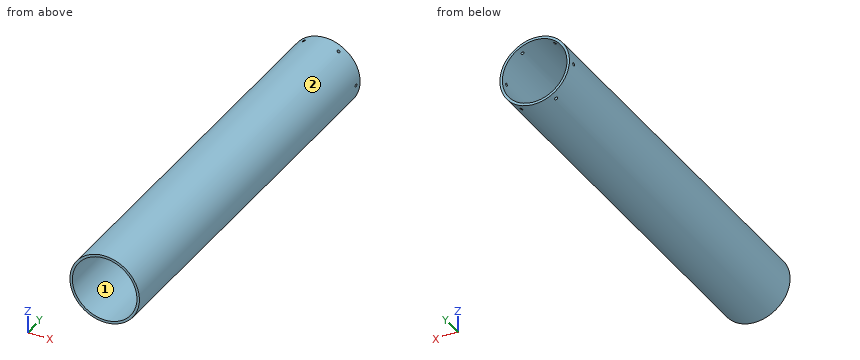
```python
from build123d import *

# Parameters (mm, degrees)
SKETCH1_R               = 70
SKETCH1_R_2             = 65
BOSS_EXTRUDE1_DEPTH     = 800
CUT_EXTRUDE1_REACH      = 808.102
CUT_EXTRUDE1_END_RADIUS = 70
SKETCH2_R               = 3.05
CIRPATTERN1_COUNT       = 6


with BuildPart() as part:
    # Sketch1 → Boss-Extrude1 (new body)
    with BuildSketch(Plane(origin=(0, 0, 0), x_dir=(1, 0, 0), z_dir=(0, 1, 0))):
        with Locations(Location((0, 0, 0), (0, 0, 270))):
            Circle(SKETCH1_R)
        with Locations(Location((0, 0, 0), (0, 0, 270))):
            Circle(SKETCH1_R_2, mode=Mode.SUBTRACT)
    extrude(amount=BOSS_EXTRUDE1_DEPTH)

    # Cut-Extrude1: up to this cylinder (the profile starts inside it)
    cut_extrude1_end = Plane(origin=(0, 785, 0), z_dir=(0, -1, 0)) * Cylinder(CUT_EXTRUDE1_END_RADIUS, 1757.204, mode=Mode.PRIVATE)
    # Sketch2 → Cut-Extrude1 (cut, up to the surface)
    with BuildSketch(Plane(origin=(0, 0, 0), x_dir=(0, 0, -1), z_dir=(1, 0, 0)), mode=Mode.PRIVATE) as cut_extrude1_sk1:
        with Locations((0, 785)):
            Circle(SKETCH2_R)
    cut_extrude1_tool1 = extrude(cut_extrude1_sk1.sketch, amount=-CUT_EXTRUDE1_REACH, mode=Mode.PRIVATE) & cut_extrude1_end
    cut_extrude1 = cut_extrude1_tool1.solids().sort_by_distance((0, 785, 0))[0]
    add(cut_extrude1, mode=Mode.SUBTRACT)

    # CirPattern1: Cut-Extrude1 ×6 about axis
    cirpattern1_axis = Axis((0, 800, 0), (0, 1, 0))
    for i in range(1, CIRPATTERN1_COUNT):
        add(cut_extrude1.rotate(cirpattern1_axis, i * 360 / CIRPATTERN1_COUNT), mode=Mode.SUBTRACT)


solid = part.part
```
Can you work these out from the model? Positions are in its coordinate system, mm. Face numbers are marked on the shaded views. Give positions to 0.01 mm unless a question says otherwise; leave off trailing zeros. Order: outer loops, then holes, each group sorted by start corner. A loop starts at its lowest first (then second) coordinate and runs counter-clockwise, first axis right, second up. Notation, with made-up numbers: M -1,25.25 L 15,25.25 A26 ccw 15,43.25 Z; hole C 32.25,11.25 d8. An arc over 180 degrees is marked long. Write item = value, one per line. Start each with the question number.
Q1. Will these pins go through, and if not, where does the flat tip stop? pin 1 Ø6 at (y, z) = (389.5, 14.5) entering from -X; pin 2 Ø12 at (y, z) = (100, 38) entering from -X; pin 3 Ø1 at (x, y) = (2.5, 522) entering from -Z.
Q2. I need wall thicknesses on probe 1 along X at (y, z) = (222, 0); probe 2 along Y at (x, z) = (67.35, 0); probe 3 along Z at (x, y) = (4.5, 317). Which ranges of each line are inside material? Lowest first, please. Write a range as [from, to].
Q3. Suppose I cut it at B-B (z = 44). Write out the boundary of the cut face in (x, y), plus the area to 3 significant figures.
Q4. Suppose I cut it at C-C (y = 682.5). Write out the boundary of the cut face in (x, z), plus the area to 3 significant figures.
Q5. Suppose I cut it at A-A (x = 0). Write out the boundary of the cut face in (y, z).
Q6. We'd pull the mould along X, two halves only. Please class the marked faces 1 and 2: pulls with the +X half, pulls with the -X half, needs draft (parallel to the pull), parting line crosses it, or undercut.
Check result:
q1.pin_1 = -69.05
q1.pin_2 = -62.26
q1.pin_3 = -69.97
q2.probe_1 = [-70, -65], [65, 70]
q2.probe_2 = [0, 781.95], [788.05, 800]
q2.probe_3 = [-69.86, -64.84], [64.84, 69.86]
q3.outline = M -54.44,0 L -47.84,0 L -47.84,800 L -54.44,800 Z; M 47.84,0 L 54.44,0 L 54.44,800 L 47.84,800 Z
q3.area = 10,600 mm2
q4.outline = C 0,0 d140; hole C 0,0 d130
q4.area = 2,120 mm2
q5.outline = M 0,-70 L 800,-70 L 800,-65 L 0,-65 Z; M 0,65 L 800,65 L 800,70 L 0,70 Z
q6.face_1 = undercut
q6.face_2 = parting line crosses it
